from build123d import *

# Parameters (mm, degrees)
EXTRUDE_1_DEPTH = 10


with BuildPart() as part:
    # 草图1 → 凸台-拉伸1 (new body, symmetric)
    with BuildSketch(Plane.XY):
        with BuildLine():
            Line((-10.5, 15), (-10.5, 0))
            Line((-10.5, 0), (10.5, 0))
            Line((10.5, 0), (10.5, 15))
            Line((10.5, 15), (9.233092656, 15))
            ThreePointArc((9.233092656, 15), (0, 9.5), (-9.233092656, 15))
            Line((-9.233092656, 15), (-10.5, 15))
        make_face()
    extrude(amount=EXTRUDE_1_DEPTH, both=True)


solid = part.part
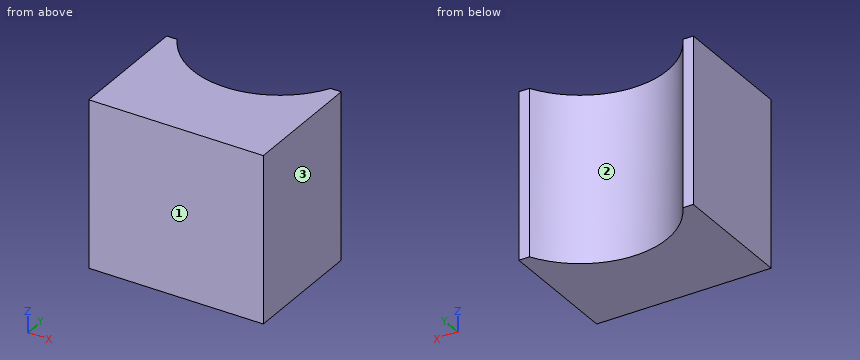
Check sheet for the modelled part. Datum: model origin and axes. Units: mm. Face numbers are marked on the shaded views. Round coordinates to 2 decimals unless told otherwise and drop trailing zeros. Order: outer loops, then holes, each group sorted by start corner. A loop starts at its lowest first (then second) coordinate and runs counter-clockwise, first axis right, second up.
(1) Scan lines: probe 1 along X at (y, z) = (10.75, 6.25); probe 2 along X at (y, z) = (12.5, -1.5); probe 3 along Y at (x, z) = (8.25, -1.5). Record each from-to range of solid material in increasing order.
(2) Draft check along X on the marked faces 1, 2 and 3. Enter one of: pulls with the +X half, pulls with the -X half, needs draft (parallel to the pull), parting line crosses it, or undercut.
(3) Cross-section at D-D, the plane x = 1.25. Enter the section's corners in (y, z).
(4) Cross-section at A-A, the plane y = 11.25. Enter the section's corners in (x, z), and give its area (3 significant figures).
(5) Cross-section at B-B, the plane z = -6.25. Enter the section's corners in (x, y), and give its area (3 significant figures).
(6) Cross-section at C-C, the plane y = 12.75. Enter the section's corners in (x, z).
(7) Go/stop test with flat-tipped pins: P1, Ø6, axis at x = 2, z = 7.5, coming from the +Y side; P2, Ø4, axis at x = -4.5, z = 0, coming from the +Y side. Record where each tip stops, or that it passes through.
Check sheet entries:
1. probe 1: x = -10.5 to -4.97, 4.97 to 10.5
1. probe 2: x = -10.5 to -7.35, 7.35 to 10.5
1. probe 3: y = 0 to 13.5
2. face 1: needs draft
2. face 2: undercut
2. face 3: pulls with the +X half
3. outline: (0, -10) - (9.57, -10) - (9.57, 10) - (0, 10) - close
4. outline: (-10.5, -10) - (-5.8, -10) - (-5.8, 10) - (-10.5, 10) - close; (5.8, -10) - (10.5, -10) - (10.5, 10) - (5.8, 10) - close
4. area: 188 mm2
5. outline: (-10.5, 0) - (10.5, 0) - (10.5, 15) - (9.23, 15) arc R10.5 cw to (-9.23, 15) - (-10.5, 15) - close
5. area: 243 mm2
6. outline: (-10.5, -10) - (-7.6, -10) - (-7.6, 10) - (-10.5, 10) - close; (7.6, -10) - (10.5, -10) - (10.5, 10) - (7.6, 10) - close
7. P1: stops at y = 10.77
7. P2: stops at y = 11.75
